Here's how the part is built. I have some questions about the finished solid (model axes, mm). Coordinates: 2 decimals unless noted, no trailing zeros. Order: outer loops, then holes, each group sorted by start corner. A loop starts at its lowest first (then second) coordinate and runs counter-clockwise, first axis right, second up. Notation, with made-up numbers: (46, 20.25) - (68, 20.25) arc R28 cw to (68, 48.25) - close; hole circle Ø5 at (-36.5, 25). An arc over 180 degrees is marked (long way). Use one line per item in the form item = value. Start each with the question number.
from build123d import *

# Parameters (mm, degrees)
SKETCH_W  = 100
SKETCH_H  = 125
SKETCH_R  = 1.5
PAD_DEPTH = 2.5
FILLET_R  = 1


with BuildPart() as part:
    # Sketch → Pad (new body)
    with BuildSketch(Plane.XY):
        Rectangle(SKETCH_W, SKETCH_H)
        with Locations((-43.75, 53.059436)):
            Circle(SKETCH_R, mode=Mode.SUBTRACT)
        with Locations((43.75, 53.059436)):
            Circle(SKETCH_R, mode=Mode.SUBTRACT)
        with Locations((43.75, 5.559436)):
            Circle(SKETCH_R, mode=Mode.SUBTRACT)
        with Locations((43.75, -14.440564)):
            Circle(SKETCH_R, mode=Mode.SUBTRACT)
        with Locations((4.75, -14.440564)):
            Circle(SKETCH_R, mode=Mode.SUBTRACT)
        with Locations((43.75, -51.640564)):
            Circle(SKETCH_R, mode=Mode.SUBTRACT)
        with Locations((-43.75, 5.559436)):
            Circle(SKETCH_R, mode=Mode.SUBTRACT)
        with Locations((4.75, -51.640564)):
            Circle(SKETCH_R, mode=Mode.SUBTRACT)
    extrude(amount=PAD_DEPTH)

    # Fillet
    fillet_edges = [part.edges().sort_by_distance(p)[0] for p in [
        (50, 62.5, 1.25),
        (50, -62.5, 1.25),
        (50, 0, 0),
        (50, 0, 2.5),
        (-50, 62.5, 1.25),
        (0, 62.5, 0),
        (0, 62.5, 2.5),
        (-50, -62.5, 1.25),
        (-50, 0, 0),
        (-50, 0, 2.5),
        (0, -62.5, 0),
        (0, -62.5, 2.5),
    ]]
    fillet(fillet_edges, radius=FILLET_R)


solid = part.part
1) If we mould it in two halves opening along X, with no side actions, what happens to faces 1 (the flat face through (-1, 1, 2.5)), 2 (the cylindrical face through (42.56, -52.553, 1.232))? For each: pulls with the +X half, pulls with the -X half, needs draft (parallel to the pull), parting line crosses it, or undercut.
2) I need wall thicknesses on probe 1 along Y at (x, z) = (-43.75, 1.3); probe 2 along Y at (x, z) = (43.75, 1.2); probe 3 along X at (y, z) = (-51.5, 0.7). Which ranges of each line are inside material? Lowest first, please. Write a range as [from, to].
3) For pin 1 (4 mm diameter, centred on x = 4.75, y = -14.44, fed in from -Z); pin 2 (2.5 mm diameter, centred on x = 43.75, y = 5.56, fed in from +Z), each with a flat end and sliding along its axis, tell me the tip position at first contact or that it passes through.
4) Suppose I cut it at A-A, the plane x = 43.75. List the corners of the cut face in (y, z) for me, then the cut area to 3 significant figures.
5) Suppose I cut it at B-B, the plane x = -43.75. List the corners of the cut face in (y, z) for me, then the cut area to 3 significant figures.
From the geometry:
q1.face_1 = needs draft
q1.face_2 = undercut
q2.probe_1 = [-62.5, 4.06], [7.06, 51.56], [54.56, 62.5]
q2.probe_2 = [-62.5, -53.14], [-50.14, -15.94], [-12.94, 4.06], [7.06, 51.56], [54.56, 62.5]
q2.probe_3 = [-49.95, 3.26], [6.24, 42.26], [45.24, 49.95]
q3.pin_1 = 0
q3.pin_2 = through
q4.outline = (-62.5, 1) arc R1 ccw to (-61.5, 0) - (-53.14, 0) - (-53.14, 2.5) - (-61.5, 2.5) arc R1 ccw to (-62.5, 1.5) - close; (-50.14, 0) - (-15.94, 0) - (-15.94, 2.5) - (-50.14, 2.5) - close; (-12.94, 0) - (4.06, 0) - (4.06, 2.5) - (-12.94, 2.5) - close; (7.06, 0) - (51.56, 0) - (51.56, 2.5) - (7.06, 2.5) - close; (54.56, 0) - (61.5, 0) arc R1 ccw to (62.5, 1) - (62.5, 1.5) arc R1 ccw to (61.5, 2.5) - (54.56, 2.5) - close
q4.area = 282 mm2
q5.outline = (-62.5, 1) arc R1 ccw to (-61.5, 0) - (4.06, 0) - (4.06, 2.5) - (-61.5, 2.5) arc R1 ccw to (-62.5, 1.5) - close; (7.06, 0) - (51.56, 0) - (51.56, 2.5) - (7.06, 2.5) - close; (54.56, 0) - (61.5, 0) arc R1 ccw to (62.5, 1) - (62.5, 1.5) arc R1 ccw to (61.5, 2.5) - (54.56, 2.5) - close
q5.area = 297 mm2
